from build123d import *

# Parameters (mm, degrees)
EXTRUDE_THIN1_DEPTH                      = 36.2
SKETCH2_W                                = 46
SKETCH2_H                                = 46
BOSS_EXTRUDE1_DEPTH                      = 4
CBORE_FOR_M4_SHCS1_D                     = 4.5
CBORE_FOR_M4_SHCS1_DEPTH                 = 6
CBORE_FOR_M4_SHCS1_CBORE_D               = 8
CBORE_FOR_M4_SHCS1_CBORE_DEPTH           = 4
CBORE_FOR_M4_SHCS1_ON_FACE_2_D           = 4.5
CBORE_FOR_M4_SHCS1_ON_FACE_2_DEPTH       = 6
CBORE_FOR_M4_SHCS1_ON_FACE_2_CBORE_D     = 8
CBORE_FOR_M4_SHCS1_ON_FACE_2_CBORE_DEPTH = 4


with BuildPart() as part:
    # Sketch1 → Extrude-Thin1 (new body)
    with BuildSketch(Plane(origin=(0, 0, 0), x_dir=(1, 0, 0), z_dir=(0, 1, 0))):
        Polygon((-40, 0), (0, 0), (0, -40), (6, -40), (6, 6), (-40, 6), align=None)
    extrude(amount=EXTRUDE_THIN1_DEPTH)

    # Sketch2 → Boss-Extrude1 (add)
    with BuildSketch(Plane(origin=(0, 36.2, 0), x_dir=(1, 0, 0), z_dir=(0, 1, 0))):
        with Locations((-17, -17)):
            Rectangle(SKETCH2_W, SKETCH2_H)
    extrude(amount=BOSS_EXTRUDE1_DEPTH)

    # CBORE for M4 SHCS1
    with Locations(Plane(origin=(6, 18.1, 20), x_dir=(0, 0, 1), z_dir=(1, 0, 0))):
        with Locations((0, 0)):
            CounterBoreHole(CBORE_FOR_M4_SHCS1_D / 2, CBORE_FOR_M4_SHCS1_CBORE_D / 2, CBORE_FOR_M4_SHCS1_CBORE_DEPTH, depth=CBORE_FOR_M4_SHCS1_DEPTH)

    # CBORE for M4 SHCS1 on face 2
    with Locations(Plane(origin=(-20, 18.1, -6), x_dir=(-1, 0, 0), z_dir=(0, 0, -1))):
        with Locations((0, 0)):
            CounterBoreHole(CBORE_FOR_M4_SHCS1_ON_FACE_2_D / 2, CBORE_FOR_M4_SHCS1_ON_FACE_2_CBORE_D / 2, CBORE_FOR_M4_SHCS1_ON_FACE_2_CBORE_DEPTH, depth=CBORE_FOR_M4_SHCS1_ON_FACE_2_DEPTH)


solid = part.part
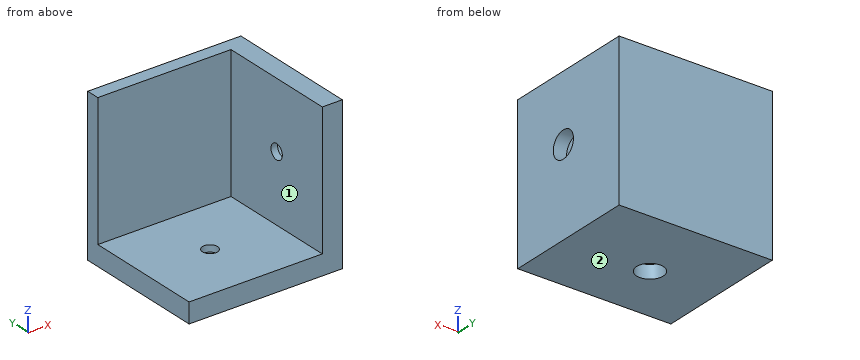
Source: CAD feature listing. Evaluate the final solid. Frame: model axes, mm. Face numbers are marked on the shaded views. A direction names the side the tool comes from. Round coordinates to 2 decimals unless told otherwise and drop trailing zeros. Loops run counter-clockwise (first coordinate to the right, second up) from the corner with the lowest first, then second, coordinate; pieces in that order, holes last. Notation, with made-up numbers: (78, 43) - (87, 43) arc R13 ccw to (87, 48) - close; hole circle Ø3 at (46.25, 78). An arc over 180 degrees is marked (long way). Write item = value, one per line. Start each with the question number.
Item 1: Reachability of the marked faces 1 and 2 from +Z, -Z, +X, -X, +Y, -Y: full face, straight path, thin tool, end or side. Return the list, or none.
Item 2: Material intervals for line 1 (Y direction, x = 3, z = 20); line 2 (Z direction, x = 2.95, y = 18.1); line 3 (Z direction, x = -14.5, y = 34.5), sorted ascending.
Item 3: Section query A-A on z = 20. Output: boundary loops of the cut face in (x, y), plus the area to 3 significant figures.
Item 4: First-contact query: pin 1 Ø1 at (x, y) = (-10.5, 34.5) entering from +Z; pin 2 Ø18 at (y, z) = (15.5, 13) entering from -X; pin 3 Ø4 at (y, z) = (20, 21.5) entering from +X; pin 4 Ø20 at (x, z) = (-18.5, 19.5) entering from -Y. Flat tips, straight axial feed; report the tip coordinate or a pass-through.
Item 5: Section query C-C on y = 18.1. Output: boundary loops of the cut face in (x, z), plus the area to 3 significant figures.
Item 6: Section query B-B on x = -20. Output: boundary loops of the cut face in (y, z), plus the area to 3 significant figures.
Item 7: Section query D-D on z = 35. Output: boundary loops of the cut face in (x, y), plus the area to 3 significant figures.
Results list:
q1.face_1 = +Z, -X, -Y
q1.face_2 = -Z, +X, -X, +Y, -Y
q2.line_1 = 0 to 14.1, 22.1 to 40.2
q2.line_2 = -6 to 16, 24 to 40
q2.line_3 = -6 to 0
q3.outline = (-40, 36.2) - (0, 36.2) - (0, 20.35) - (2, 20.35) - (2, 22.1) - (6, 22.1) - (6, 40.2) - (-40, 40.2) - close; (0, 0) - (6, 0) - (6, 14.1) - (2, 14.1) - (2, 15.85) - (0, 15.85) - close
q3.area = 360 mm²
q4.pin_1 = 0
q4.pin_2 = 0
q4.pin_3 = 6
q4.pin_4 = 36.2
q5.outline = (-40, -6) - (-24, -6) - (-24, -2) - (-22.25, -2) - (-22.25, 0) - (-40, 0) - close; (-17.75, -2) - (-16, -2) - (-16, -6) - (6, -6) - (6, 16) - (2, 16) - (2, 17.75) - (0, 17.75) - (0, 0) - (-17.75, 0) - close; (0, 22.25) - (2, 22.25) - (2, 24) - (6, 24) - (6, 40) - (0, 40) - close
q5.area = 434 mm²
q6.outline = (0, -6) - (14.1, -6) - (14.1, -2) - (15.85, -2) - (15.85, 0) - (0, 0) - close; (20.35, -2) - (22.1, -2) - (22.1, -6) - (40.2, -6) - (40.2, 40) - (36.2, 40) - (36.2, 0) - (20.35, 0) - close
q6.area = 360 mm²
q7.outline = (-40, 36.2) - (0, 36.2) - (0, 0) - (6, 0) - (6, 40.2) - (-40, 40.2) - close
q7.area = 401 mm²
